```python
from build123d import *

# Parameters (mm, degrees)
CBORE_FOR_M3_HEX_HEAD_MACHINE_SCREW1_AT_COUNT = 2
CBORE_FOR_M3_HEX_HEAD_MACHINE_SCREW1_AT_PITCH = 21.213203436
CBORE_FOR_M3_HEX_HEAD_MACHINE_SCREW1_2_COUNT  = 2
CBORE_FOR_M3_HEX_HEAD_MACHINE_SCREW1_2_PITCH  = 21.213203436
CBORE_FOR_M3_HEX_HEAD_MACHINE_SCREW1_3_COUNT  = 2
CBORE_FOR_M3_HEX_HEAD_MACHINE_SCREW1_3_PITCH  = 30


with BuildPart() as part:
    # Sketch1 → Revolve1 (revolve)
    with BuildSketch(Plane.XY, mode=Mode.PRIVATE) as revolve1_sk:
        Polygon((21.35, 0), (21.35, 5), (3.048, 5), (3.048, 1), (4, 1), (4, 0), align=None)
    revolve(revolve1_sk.sketch.rotate(Axis((0, 0, 0), (0, 1, 0)), 90), axis=Axis((0, 0, 0), (0, 1, 0)))

    # Sketch3 → CBORE for M3 Hex Head Machine Screw1 (revolve, cut)
    with BuildSketch(Plane(origin=(4.590221075, 5, -14.280401622), x_dir=(0, 0, 1), z_dir=(1, 0, 0))):
        Polygon((0, 0), (0, 5), (1.7, 5), (1.7, 2.3), (4.2, 2.3), (4.2, 0.025), (4.225, 0), align=None)
    cbore_for_m3_hex_head_machine_screw1 = revolve(axis=Axis((4.590221075, 11.35, -14.280401622), (0, -1, 0)), mode=Mode.SUBTRACT)

    # CBORE for M3 Hex Head Machine Screw1 at: CBORE for M3 Hex Head Machine Screw1 ×2
    with Locations(*[Vector(-0.8895696849339428, 0, 0.4567994917319041) * (i * CBORE_FOR_M3_HEX_HEAD_MACHINE_SCREW1_AT_PITCH) for i in range(1, CBORE_FOR_M3_HEX_HEAD_MACHINE_SCREW1_AT_COUNT)]):
        add(cbore_for_m3_hex_head_machine_screw1, mode=Mode.SUBTRACT)

    # CBORE for M3 Hex Head Machine Screw1 2: CBORE for M3 Hex Head Machine Screw1 ×2
    with Locations(*[Vector(0.4567994917319041, 0, 0.8895696849339427) * (i * CBORE_FOR_M3_HEX_HEAD_MACHINE_SCREW1_2_PITCH) for i in range(1, CBORE_FOR_M3_HEX_HEAD_MACHINE_SCREW1_2_COUNT)]):
        add(cbore_for_m3_hex_head_machine_screw1, mode=Mode.SUBTRACT)

    # CBORE for M3 Hex Head Machine Screw1 3: CBORE for M3 Hex Head Machine Screw1 ×2
    with Locations(*[Vector(-0.3060147383085738, 0, 0.9520267748009691) * (i * CBORE_FOR_M3_HEX_HEAD_MACHINE_SCREW1_3_PITCH) for i in range(1, CBORE_FOR_M3_HEX_HEAD_MACHINE_SCREW1_3_COUNT)]):
        add(cbore_for_m3_hex_head_machine_screw1, mode=Mode.SUBTRACT)


solid = part.part
```
Input: part model. Units: mm. Frame: model coordinates. A direction names the side the tool comes from. Coordinates: 2 decimals unless noted, no trailing zeros. Loops run counter-clockwise (first coordinate to the right, second up) from the corner with the lowest first, then second, coordinate; pieces in that order, holes last. Notation, with made-up numbers: M 42.5,-12.5 L 64.5,-12.5 A6 ccw 64.5,-4.5 Z; hole C -13.75,73.25 d10. An arc over 180 degrees is marked long. Answer in a Markdown table with one row per item.
1. Section A-A, the plane y = 4.1. Output: boundary loops of the cut face in (x, z), then the cut area to 3 significant figures.
Response:
| item | result |
|---|---|
| outline | C 0,0 d42.7; hole C -14.28,-4.59 d8.4; hole C -4.59,14.28 d8.4; hole C 0,0 d6.1; hole C 4.59,-14.28 d8.4; hole C 14.28,4.59 d8.4 |
| area | 1,180 mm2 |
2. Material intervals for line 1 (X direction, y = 3.4, z = 1.5); line 2 (X direction, y = 4.15, z = 0); line 3 (Z direction, x = -6, y = 4.1), sorted ascending.
Response:
| item | result |
|---|---|
| line 1 | x = -21.3 to -2.65, 2.65 to 11.44, 17.12 to 21.3 |
| line 2 | x = -21.35 to -3.05, 3.05 to 21.35 |
| line 3 | z = -20.49 to 10.32, 18.24 to 20.49 |
3. First-contact query: pin 1 (5 mm diameter, centred on x = 14.28, z = 4.59, fed in from +Y); pin 2 (2 mm diameter, centred on y = 2, z = -15.5, fed in from -X); pin 3 (1 mm diameter, centred on y = 1.5, z = -3.5, fed in from -X). Flat tips, straight axial feed; report the tip coordinate or a pass-through.
Response:
| item | result |
|---|---|
| pin 1 | stops at y = 2.7 |
| pin 2 | stops at x = -15.67 |
| pin 3 | stops at x = -21.14 |
4. Reachability of faces 1 (the cylindrical face through (5.24, 1.37, -12.71)), 2 (the cylindrical face through (4.406, 3.853, -18.476)), 3 (the cylindrical face through (3.905, 0.493, 0.867)) from +Z, -Z, +X, -X, +Y, -Y: full face, straight path, thin tool, end or side. Return the list, or none.
Response:
| item | result |
|---|---|
| face 1 | +Y, -Y |
| face 2 | +Y |
| face 3 | -Y |
5. Draft query along Z for faces 4 (the flat face through (4.4, 0, -0.3)), 5 (the cylindrical face through (18.94, 2.54, -9.85)), 6 (the cylindrical face through (-15.966, 1.369, -4.812)). Return one class per face: pulls with the +Z half, pulls with the -Z half, needs draft (parallel to the pull), parting line crosses it, or undercut.
Response:
| item | result |
|---|---|
| face 4 | needs draft |
| face 5 | parting line crosses it |
| face 6 | undercut |
